from build123d import *

# Parameters (mm, degrees)
F1_DEPTH = 45.466
F2_DEPTH = 25.4
F4_DEPTH = 46.736


with BuildPart() as f1:
    # F0 (on Front) → F1 (new body)
    with BuildSketch(Plane.XZ):
        with BuildLine():
            ThreePointArc((-36.8620457054, 0), (-26.0654024867, 26.0654024867), (0, 36.8620457054))
            Line((0, 36.8620457054), (0, 57.9813979566))
            Line((0, 57.9813979566), (-68.4616416693, 57.9813979566))
            Line((-68.4616416693, 57.9813979566), (-68.4616416693, 0))
            Line((-68.4616416693, 0), (-51.4429248869, 0))
            Line((-51.4429248869, 0), (-36.8620457054, 0))
        make_face()
        with BuildLine():
            ThreePointArc((0, -36.8620457054), (-26.0654024867, -26.0654024867), (-36.8620457054, 0))
            Line((-36.8620457054, 0), (-51.4429248869, 0))
            Line((-51.4429248869, 0), (-51.4429248869, -49.0166470408))
            Line((-51.4429248869, -49.0166470408), (0, -49.0166470408))
            Line((0, -49.0166470408), (0, -36.8620457054))
        make_face()
    extrude(amount=F1_DEPTH)

    # F0 (on Front) → F2 (join)
    with BuildSketch(Plane.XZ):
        with BuildLine():
            Line((28.4934528172, 0), (36.8620457054, 0))
            ThreePointArc((36.8620457054, 0), (36.3777391302, 5.9557123304), (34.9375453863, 11.7549281567))
            Line((34.9375453863, 11.7549281567), (0, 11.7549281567))
            Line((0, 11.7549281567), (0, 0))
            Line((0, 0), (28.4934528172, 0))
        make_face()
        with BuildLine():
            ThreePointArc((28.4934528172, -23.3866107023), (34.7068968192, -12.4194092761), (36.8620457054, 0))
            Line((36.8620457054, 0), (28.4934528172, 0))
            Line((28.4934528172, 0), (28.4934528172, -23.3866107023))
        make_face()
        with BuildLine():
            ThreePointArc((34.9375453863, 11.7549281567), (36.3777391302, 5.9557123304), (36.8620457054, 0))
            Line((36.8620457054, 0), (69.7509273887, 0))
            Line((69.7509273887, 0), (69.7509273887, 11.7549281567))
            Line((69.7509273887, 11.7549281567), (34.9375453863, 11.7549281567))
        make_face()
        with BuildLine():
            Line((0, 11.7549281567), (34.9375453863, 11.7549281567))
            ThreePointArc((34.9375453863, 11.7549281567), (21.5116214476, 29.9342705988), (0, 36.8620457054))
            Line((0, 36.8620457054), (0, 11.7549281567))
        make_face()
        with BuildLine():
            Line((28.4934528172, -32.1296229959), (28.4934528172, -23.3866107023))
            ThreePointArc((28.4934528172, -23.3866107023), (23.6882112756, -28.2432126387), (18.0692484551, -32.1296229959))
            Line((18.0692484551, -32.1296229959), (28.4934528172, -32.1296229959))
        make_face()
        with BuildLine():
            ThreePointArc((18.0692484551, -32.1296229959), (23.6882112756, -28.2432126387), (28.4934528172, -23.3866107023))
            Line((28.4934528172, -23.3866107023), (28.4934528172, 0))
            Line((28.4934528172, 0), (0, 0))
            Line((0, 0), (0, -32.1296229959))
            Line((0, -32.1296229959), (18.0692484551, -32.1296229959))
        make_face()
        with BuildLine():
            Line((0, 11.7549281567), (0, 36.8620457054))
            ThreePointArc((0, 36.8620457054), (-26.0654024867, 26.0654024867), (-36.8620457054, 0))
            Line((-36.8620457054, 0), (0, 0))
            Line((0, 0), (0, 11.7549281567))
        make_face()
        with BuildLine():
            ThreePointArc((-36.8620457054, 0), (-26.0654024867, 26.0654024867), (0, 36.8620457054))
            Line((0, 36.8620457054), (0, 57.9813979566))
            Line((0, 57.9813979566), (-68.4616416693, 57.9813979566))
            Line((-68.4616416693, 57.9813979566), (-68.4616416693, 0))
            Line((-68.4616416693, 0), (-51.4429248869, 0))
            Line((-51.4429248869, 0), (-36.8620457054, 0))
        make_face()
        with BuildLine():
            ThreePointArc((0, -36.8620457054), (9.3393463962, -35.6593188729), (18.0692484551, -32.1296229959))
            Line((18.0692484551, -32.1296229959), (0, -32.1296229959))
            Line((0, -32.1296229959), (0, -36.8620457054))
        make_face()
        with BuildLine():
            Line((0, -32.1296229959), (0, 0))
            Line((0, 0), (-36.8620457054, 0))
            ThreePointArc((-36.8620457054, 0), (-26.0654024867, -26.0654024867), (0, -36.8620457054))
            Line((0, -36.8620457054), (0, -32.1296229959))
        make_face()
        with BuildLine():
            ThreePointArc((0, -36.8620457054), (-26.0654024867, -26.0654024867), (-36.8620457054, 0))
            Line((-36.8620457054, 0), (-51.4429248869, 0))
            Line((-51.4429248869, 0), (-51.4429248869, -49.0166470408))
            Line((-51.4429248869, -49.0166470408), (0, -49.0166470408))
            Line((0, -49.0166470408), (0, -36.8620457054))
        make_face()
    extrude(amount=F2_DEPTH)

    # F3 (on Right) → F4 (join)
    with BuildSketch(Plane.YZ):
        with BuildLine():
            ThreePointArc((18.8913277671, -26.0016833187), (28.6368136719, -14.5911857958), (32.1398475449, 0))
            ThreePointArc((32.1398475449, 0), (31.7441526763, 5.0277799349), (30.5668113916, 9.9317592377))
            ThreePointArc((30.5668113916, 9.9317592377), (18.8913283341, 26.0016829067), (0, 32.1398475449))
            ThreePointArc((0, 32.1398475449), (-18.8913281553, 26.0016830366), (-30.566811255, 9.9317596581))
            ThreePointArc((-30.566811255, 9.9317596581), (-30.5668114341, -9.9317591071), (-18.8913278804, -26.0016832363))
            ThreePointArc((-18.8913278804, -26.0016832363), (-7e-08, -32.1398475449), (18.8913277671, -26.0016833187))
        make_face()
        with BuildLine():
            ThreePointArc((30.5668113916, 9.9317592377), (31.7441526763, 5.0277799349), (32.1398475449, 0))
            ThreePointArc((32.1398475449, 0), (28.6368136719, -14.5911857958), (18.8913277671, -26.0016833187))
            Line((18.8913277671, -26.0016833187), (37.7826567956, -12.2763293689))
            Line((37.7826567956, -12.2763293689), (30.5668113916, 9.9317592377))
        make_face()
        with BuildLine():
            ThreePointArc((0, 32.1398475449), (18.8913283341, 26.0016829067), (30.5668113916, 9.9317592377))
            Line((30.5668113916, 9.9317592377), (23.350966085, 32.1398475449))
            Line((23.350966085, 32.1398475449), (0, 32.1398475449))
        make_face()
        with BuildLine():
            Line((0, -39.7270363519), (18.8913277671, -26.0016833187))
            ThreePointArc((18.8913277671, -26.0016833187), (-7e-08, -32.1398475449), (-18.8913278804, -26.0016832363))
            Line((-18.8913278804, -26.0016832363), (0, -39.7270363519))
        make_face()
        with BuildLine():
            ThreePointArc((-30.566811255, 9.9317596581), (-18.8913281553, 26.0016830366), (0, 32.1398475449))
            Line((0, 32.1398475449), (-23.350966085, 32.1398475449))
            Line((-23.350966085, 32.1398475449), (-30.566811255, 9.9317596581))
        make_face()
        with BuildLine():
            Line((-37.7826567956, -12.2763293689), (-18.8913278804, -26.0016832363))
            ThreePointArc((-18.8913278804, -26.0016832363), (-30.5668114341, -9.9317591071), (-30.566811255, 9.9317596581))
            Line((-30.566811255, 9.9317596581), (-37.7826567956, -12.2763293689))
        make_face()
    extrude(amount=-F4_DEPTH)


solid = f1.part
For this review, take the finished solid that the model builds, in its own axes (mm). A direction names the side the tool comes from. Round coordinates to 2 decimals unless told otherwise and drop trailing zeros. Loops run counter-clockwise (first coordinate to the right, second up) from the corner with the lowest first, then second, coordinate; pieces in that order, holes last. Notation, with made-up numbers: (28, 2.5) - (78, 2.5) arc R12 cw to (78, 21.5) - close; hole circle Ø1 at (74.5, 17). An arc over 180 degrees is marked (long way). Answer as CSV lines item,"result".
(1) Mouldability with a two-part tool opening along Z and no side actions: class faces 1 (the face through (19, -25.4, 1)), 2 (the face through (0.3, 0, 12.7)), 3 (the face through (9.211, -12.522, -35.693)), 4 (the face through (-34, -22, 57.981)) as +Z half, -Z half, draft (parallel to the pull), parting line (faces both ways), or undercut.
Checked values:
face 1,"undercut"
face 2,"draft"
face 3,"-Z half"
face 4,"+Z half"
(2) Consider section C-C on y = -35.5. Give the boundary of the cut face in (x, z), then the cut area to 3 significant figures.
Checked values:
outline,"(-68.46, 0) - (-51.44, 0) - (-51.44, -49.02) - (0, -49.02) - (0, -36.86) arc R36.86 cw to (-34.13, -13.93) - (0, -13.93) - (0, -5.25) - (-36.49, -5.25) arc R36.86 cw to (0, 36.86) - (0, 57.98) - (-68.46, 57.98) - close"
area,"4,660 mm2"
(3) Tool access review of faces 5 (the face through (-46.736, 14, -3)), 6 (the face through (-60, -22, 0)), 7 (the face through (0, -22, 47)): name each direction out of +Z, -Z, +X, -X, +Y, -Y from which nothing blocks a thin tool from reaching the whole face with its end or side.
Checked values:
face 5,"+Z, -Z, -X, +Y"
face 6,"-Z, -X, +Y, -Y"
face 7,"+Z, +X, +Y, -Y"
(4) Consider section B-B on z = -19.5. Give the boundary of the cut face in (x, y), then the cut area to 3 significant figures.
Checked values:
outline,"(-51.44, -45.47) - (-31.28, -45.47) - (-31.28, -27.84) - (0, -27.84) - (0, -25.4) - (31.28, -25.4) - (31.28, 0) - (0, 0) - (0, 27.84) - (-46.74, 27.84) - (-46.74, 0) - (-51.44, 0) - close"
area,"3,880 mm2"
(5) Insertion check: P1, Ø2.5, axis at y = -10, z = -27, coming from the +X side; P2, Ø5, axis at y = -5.5, z = -15.5, coming from the +X side; P3, Ø1, axis at x = 21, z = -33.5, coming from the -Y side; P4, Ø24.5, axis at y = 12.5, z = 10.5, coming from the +X side. Each pin has a flat end and moves straight along its axis. Give the tip position at first contact, or say it passes through.
Checked values:
P1,"stops at x = 28.49"
P2,"stops at x = 34.49"
P3,"passes through"
P4,"stops at x = 0"
(6) Wall thickness on line 1 (X direction, y = -15, z = -25); line 2 (Y direction, x = 17, z = -19); line 3 (X direction, y = -38.5, z = 46): over which ranges is each line inside the solid? List them lowest first.
Checked values:
line 1,"x = -51.44 to 28.49"
line 2,"y = -25.4 to 0"
line 3,"x = -68.46 to 0"
(7) Consider section D-D on y = 28. Give the boundary of the cut face in (x, z), then the cut area to 3 significant figures.
Checked values:
outline,"(-46.74, -19.38) - (0, -19.38) - (0, 17.83) - (-46.74, 17.83) - close"
area,"1,740 mm2"
(8) Consider section A-A on y = -17. Give the boundary of the cut face in (x, z).
Checked values:
outline,"(-68.46, 0) - (-51.44, 0) - (-51.44, -49.02) - (0, -49.02) - (0, -36.86) arc R36.86 ccw to (18.07, -32.13) - (28.49, -32.13) - (28.49, -23.39) arc R36.86 ccw to (36.86, 0) - (69.75, 0) - (69.75, 11.75) - (34.94, 11.75) arc R36.86 ccw to (0, 36.86) - (0, 57.98) - (-68.46, 57.98) - close"
